```python
from build123d import *

# Parameters (mm, degrees)
BOSS_EXTRUDE1_DEPTH = 12.7
BOSS_EXTRUDE2_DEPTH = 38.1
SKETCH4_R           = 12.7
SKETCH4_R_2         = 5.08
CUT_EXTRUDE1_DEPTH  = 51.8
SKETCH3_R           = 5.18795
CUT_EXTRUDE2_DEPTH  = 13.7
FILLET1_R           = 2.54


with BuildPart() as part:
    # Sketch1 → Boss-Extrude1 (new body)
    with BuildSketch(Plane.XY):
        with BuildLine():
            Line((-44.45, -12.7), (-44.45, -38.1))
            ThreePointArc((-44.45, -38.1), (0, -82.55), (44.45, -38.1))
            Line((44.45, -38.1), (44.45, -12.7))
            Line((44.45, -12.7), (-44.45, -12.7))
        make_face()
        Polygon((-50.8, -12.7), (-44.45, -12.7), (44.45, -12.7), (50.8, -12.7), (50.8, 0), (-50.8, 0), align=None)
    extrude(amount=BOSS_EXTRUDE1_DEPTH)

    # Sketch1_4 → Boss-Extrude2 (add)
    with BuildSketch(Plane.XY):
        Polygon((-50.8, -12.7), (-44.45, -12.7), (44.45, -12.7), (50.8, -12.7), (50.8, 0), (-50.8, 0), align=None)
    extrude(amount=-BOSS_EXTRUDE2_DEPTH)

    # Sketch4 → Cut-Extrude1 (cut, through all)
    with BuildSketch(Plane.XY.offset(12.7)):
        with Locations((0, -38.1)):
            Circle(SKETCH4_R)
        with Locations((-31.75, -38.1)):
            Circle(SKETCH4_R_2)
        with Locations((31.75, -38.1)):
            Circle(SKETCH4_R_2)
        with Locations((0, -69.85)):
            Circle(SKETCH4_R_2)
    extrude(amount=-CUT_EXTRUDE1_DEPTH, mode=Mode.SUBTRACT)

    # Sketch3 → Cut-Extrude2 (cut, through all)
    with BuildSketch(Plane.XZ.offset(12.7)):
        with Locations((-31.75, -19.05)):
            Circle(SKETCH3_R)
        with Locations((31.75, -19.05)):
            Circle(SKETCH3_R)
    extrude(amount=-CUT_EXTRUDE2_DEPTH, mode=Mode.SUBTRACT)

    # Fillet1
    fillet1_edges = [part.edges().sort_by_distance(p)[0] for p in [
        (-44.45, -12.7, 6.35),
        (44.45, -12.7, 6.35),
        (0, -12.7, 0),
    ]]
    fillet(fillet1_edges, radius=FILLET1_R)


solid = part.part
```
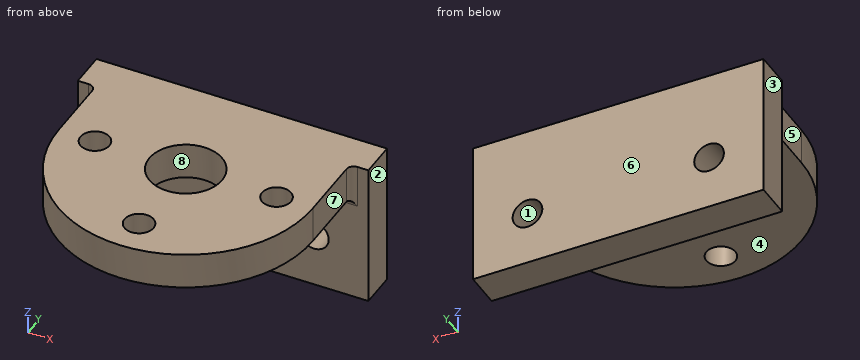
Here's how the part is built. I have some questions about the finished solid (model axes, mm). Face numbers are marked on the shaded views. A direction names the side the tool comes from. Give positions to 0.01 mm unless a question says otherwise; leave off trailing zeros. Write each loop counter-clockwise with the first axis right and the second up, starting at its lowest first coordinate (ties: lowest second). Pieces come first, ordered by that corner, then holes. Notation, with made-up numbers: M 47,-28 L 75,-28 A18 ccw 75,-6 Z; hole C 19,12 d8. An arc over 180 degrees is marked long. Put each result on its own line as item: value. Start each with the question number.
Item 1: Thinking about a two-plate mould opening in X: for the marked faces 1, 2 and 3, which applies, +X half, -X half, draft (parallel to the pull), parting line (faces both ways), or undercut?
Item 2: If we section it at C-C, the plane x = 9.5: Write out the boundary of the cut face in (y, z).
Item 3: If we section it at B-B, the plane y = -69.85: Write out the boundary of the cut face in (x, z), then the cut area to 3 significant figures.
Item 4: If we section it at D-D, the plane z = 9: Write out the boundary of the cut face in (x, y), then the cut area to 3 significant figures.
Item 5: On a 3-axis mill with a long thin cutter (end or side, diameter ignored), from which of +Z, -Z, +X, -X, +Y, -Y can I reach the whole of each face in a straight line? I mean the marked faces 4, 5, 6, 7 and 8. Say none if no direction works.
Item 6: I need wall thicknesses on L1, parallel to Y at x = 0, z = 9.75; L2, parallel to X at y = -2, z = -19; L3, parallel to X at y = -38, z = 7. Which ranges of each line are inside material? Lowest first, please. Write a range as from..to.
Item 7: If we section it at A-A, the plane z = -23: Write out the boundary of the cut face in (x, y).
Item 8: Will these pins go through, and if not, where does the flat tip stop? pin 1 (11.5 mm diameter, centred on x = -31.75, y = -38.1, fed in from -Z); pin 2 (1.5 mm diameter, centred on x = -35.5, z = -16.5, fed in from -Y); pin 3 (1 mm diameter, centred on x = -1, z = -2, fed in from -Y).
Values:
1. face 1: undercut
1. face 2: +X half
1. face 3: -X half
2. outline: M -81.52,0 L -46.53,0 L -46.53,12.7 L -81.52,12.7 Z; M -29.67,0 L -15.24,0 A2.54 cw -12.7,-2.54 L -12.7,-38.1 L 0,-38.1 L 0,12.7 L -29.67,12.7 Z
3. outline: M -31.11,0 L -5.08,0 L -5.08,12.7 L -31.11,12.7 Z; M 5.08,0 L 31.11,0 L 31.11,12.7 L 5.08,12.7 Z
3. area: 661 mm²
4. outline: M -50.8,-12.7 L -46.99,-12.7 A2.54 cw -44.45,-15.24 L -44.45,-38.1 A44.45 ccw 44.45,-38.1 L 44.45,-15.24 A2.54 cw 46.99,-12.7 L 50.8,-12.7 L 50.8,0 L -50.8,0 Z; hole C -31.75,-38.1 d10.16; hole C 0,-38.1 d25.4; hole C 0,-69.85 d10.16; hole C 31.75,-38.1 d10.16
4. area: 5,900 mm²
5. face 4: -Z, +X, -X, -Y
5. face 5: +Z, -Z, -X, -Y
5. face 6: +Z, -Z, +X, -X, +Y
5. face 7: +Z, -Z, +X, -Y
5. face 8: +Z, -Z
6. L1: -82.55..-74.93, -64.77..-50.8, -25.4..0
6. L2: -50.8..-36.94, -26.56..26.56, 36.94..50.8
6. L3: -44.45..-36.83, -26.67..-12.7, 12.7..26.67, 36.83..44.45
7. outline: M -50.8,-12.7 L -35.11,-12.7 L -35.11,0 L -50.8,0 Z; M -28.39,-12.7 L 28.39,-12.7 L 28.39,0 L -28.39,0 Z; M 35.11,-12.7 L 50.8,-12.7 L 50.8,0 L 35.11,0 Z
8. pin 1: z = 0
8. pin 2: y = -12.7
8. pin 3: y = -12.92
